Autodesk Inventor part; units mm, degrees
ref_plane "YZ Plane" through (0, 0, 0) normal (1, 0, 0) x (0, 1, 0)
ref_plane "XZ Plane" through (0, 0, 0) normal (0, 1, 0) x (-1, 0, 0)
ref_plane "XY Plane" through (0, 0, 0) normal (0, 0, 1) x (1, 0, 0)
sketch "Sketch1" plane through (0, 0, 0) normal (1, 0, 0) x (0, 1, 0)
  line L0 (0, 0) -> (45.3157, 0)
  line L1 (0, 172.72) -> (163.576, 172.72)
  line L2 (163.576, 172.72) -> (163.576, 198.12)
  line L3 (163.576, 198.12) -> (0, 198.12)
  line L4 (0, 198.12) -> (0, 172.72)
  dimension "d0" = 345.44
  dimension "d1" = 163.576
  dimension "d2" = 25.4
extrude "Extrusion1" add sketch "Sketch1" along normal blind 12.7
sketch "Sketch3" plane through (12.7, 0, 0) normal (1, 0, 0) x (0, 0, -1)
  circle A0 centre (-185.42, 146.05) radius 3.175
  line L0 (-172.72, 0) -> (-172.72, 163.576)
  line L1 (-198.12, 0) -> (-172.72, 0)
  point P0 (0, 0)
  dimension "d10" = 6.35
  dimension "d11" = 12.7
  dimension "d62" = 146.05
extrude "Extrusion3" cut sketch "Sketch3" against normal blind 25.4
chamfer "Chamfer1" distance 9.525 angle 45 1 edges at (6.35, 0, 172.72)
sketch "Sketch4" plane through (12.7, 0, 0) normal (1, 0, 0) x (0, 0, -1)
  circle A0 centre (-185.42, 146.05) radius 3.175
  circle A1 centre (-185.42, 146.05) radius 9.525
  point P0 (0, 0)
  dimension "d18" = 19.05
extrude "Extrusion4" add sketch "Sketch4" along normal blind 19.05
mirror "Mirror2" about plane through (0, 0, 0) normal (0, 0, 1) of "Extrusion1", "Extrusion3", "Chamfer1", "Extrusion4"
sketch "Sketch5" plane through (0, 0, 0) normal (-1, 0, 0) x (0, 0, 1)
  line L0 (172.72, 163.576) -> (198.12, 163.576)
  line L1 (198.12, 163.576) -> (-198.12, 163.576)
  line L2 (-198.12, 163.576) -> (-198.12, 227.076)
  line L3 (-198.12, 227.076) -> (198.12, 227.076)
  line L4 (198.12, 227.076) -> (198.12, 163.576)
  point P0 (0, 0)
  dimension "d21" = 63.5
extrude "Extrusion5" add sketch "Sketch5" against normal up to surface (12.7 mm away)
fillet "Fillet2" radius 25.4 2 edges at (6.35, 227.076, 198.12) (6.35, 227.076, -198.12)
sketch "Sketch6" plane through (12.7, 0, 0) normal (1, 0, 0) x (0, 0, -1)
  line L0 (188.595, 120.65) -> (182.245, 120.65)
  line L1 (179.07, 123.825) -> (179.07, 168.275)
  line L2 (182.245, 171.45) -> (188.595, 171.45)
  line L3 (191.77, 168.275) -> (191.77, 123.825)
  circle A0 centre (185.42, 146.05) radius 3.175
  line L4 (191.77, 120.65) -> (179.07, 171.45) construction
  line L5 (179.07, 120.65) -> (191.77, 171.45) construction
  arc A1 (182.245, 171.45) -> (179.07, 168.275) centre (182.245, 168.275) ccw
  arc A2 (191.77, 168.275) -> (188.595, 171.45) centre (188.595, 168.275) ccw
  arc A3 (188.595, 120.65) -> (191.77, 123.825) centre (188.595, 123.825) ccw
  arc A4 (179.07, 123.825) -> (182.245, 120.65) centre (182.245, 123.825) ccw
  circle A5 centre (185.42, 146.05) radius 9.525
  circle A6 centre (185.42, 165.1) radius 2.6289
  line L6 (185.42, 165.1) -> (185.42, 171.45)
  circle A7 centre (185.42, 127) radius 2.6289
  line L7 (185.42, 127) -> (185.42, 120.65)
  point P0 (0, 0)
  point P1 (191.77, 138.9505)
  point P2 (179.07, 138.9505)
  point P3 (179.07, 153.1495)
  point P4 (191.77, 153.1495)
  dimension "d25" = 12.7
  dimension "d26" = 50.8
  dimension "d27" = 3.175
  dimension "d28" = 5.2578
  dimension "d29" = 6.35
  dimension "d30" = 5.2578
  dimension "d31" = 6.35
extrude "Extrusion6" add sketch "Sketch6" along normal blind 19.05 contours L0 A4 L1 A5 L3 A3 | A5 L1 A1 L2 A2 L3
sketch "Sketch9" plane through (0, 227.076, 172.72) normal (0, 1, 0) x (1, 0, 0)
  line L0 (0, 345.44) -> (0, 0)
  line L1 (0, 228.6) -> (6.35, 228.6)
  line L2 (6.35, 228.6) -> (6.35, 116.84)
  line L3 (6.35, 116.84) -> (12.7, 116.84)
  line L4 (12.7, 345.44) -> (12.7, 0)
  line L5 (0, -25.4) -> (12.7, -25.4)
  point P0 (0, 172.72)
  point P1 (6.35, 172.72)
  point P2 (0, 172.72)
  dimension "d47" = 6.35
  dimension "d48" = 254
sketch "Sketch10" plane through (12.7, 0, 0) normal (1, 0, 0) x (0, 0, -1)
  circle A0 centre (179.07, 17.4625) radius 2.0828
  circle A1 centre (191.77, 48.4187) radius 2.0828
  circle A2 centre (179.07, 79.375) radius 2.0828
  line L0 (185.42, 0) -> (198.12, 0)
  line L1 (198.12, 88.9) -> (198.12, 0)
  line L2 (172.72, 88.9) -> (198.12, 88.9)
  line L3 (172.72, 88.9) -> (172.72, 12.7)
  line L4 (172.72, 12.7) -> (185.42, 0)
  point P0 (0, 0)
  point P1 (-12.7, 88.9)
  dimension "d49" = 6.35
  dimension "d50" = 9.525
  dimension "d51" = 25.4
  dimension "d52" = 76.2
  dimension "d53" = 88.9
  dimension "d54" = 12.7
  dimension "d55" = 4.7625
  dimension "d56" = 6.35
  dimension "d57" = 19.05
  dimension "d58" = 40.4813
  dimension "d59" = 4.1656
extrude "Extrusion8" cut sketch "Sketch10" against normal through all contours A0 | A1 | A2
mirror "Mirror3" about plane through (0, 0, 0) normal (0, 0, 1) of "Extrusion8"
sketch "Sketch11" plane through (31.75, 146.05, 185.42) normal (1, 0, 0) x (0, 0, -1)
  circle A0 centre (0, 0) radius 9.525
  circle A1 centre (0, 0) radius 3.175
  point P0 (185.42, -146.05)
extrude "Extrusion9" cut sketch "Sketch11" against normal up to surface (19.05 mm away)
sketch "Sketch12" plane through (12.7, 0, 0) normal (1, 0, 0) x (0, 0, -1)
  circle A0 centre (-185.42, 146.05) radius 3.175
  line L0 (-185.42, 165.1) -> (-185.42, 127)
  circle A1 centre (-185.42, 165.1) radius 2.6035
  circle A2 centre (-185.42, 127) radius 2.6035
  point P0 (0, 0)
  dimension "d65" = 38.1
  dimension "d66" = 5.207
  dimension "d67" = 5.207
extrude "Extrusion10" cut sketch "Sketch12" against normal blind 25.4 contours A2 | A1
sketch "Sketch13" plane through (0, 0, 0) normal (-1, 0, 0) x (0, 0, 1)
  line L0 (-60.6806, 180.6448) -> (-117.602, 180.6448)
  line L1 (-117.602, 180.6448) -> (-117.602, 215.5698)
  line L2 (-117.602, 215.5698) -> (-60.6806, 215.5698)
  line L3 (-60.6806, 215.5698) -> (-60.6806, 180.6448)
  line L4 (-60.6806, 180.6448) -> (-117.602, 215.5698) construction
  line L5 (-117.602, 180.6448) -> (-60.6806, 215.5698) construction
  line L6 (-198.12, 201.676) -> (-198.12, 0)
  line L7 (-90.0938, 214.5284) -> (-90.0938, 179.6034)
  line L8 (172.72, 227.076) -> (-172.72, 227.076)
  line L9 (-90.0938, 214.5284) -> (-28.448, 214.5284)
  line L10 (-28.448, 214.5284) -> (-28.448, 179.6034)
  line L11 (-28.448, 179.6034) -> (-90.0938, 179.6034)
  line L12 (-90.0938, 179.6034) -> (-90.0938, 214.5284)
  line L13 (-60.6806, 215.5698) -> (4.6736, 215.5698)
  line L14 (4.6736, 215.5698) -> (4.6736, 180.6448)
  line L15 (4.6736, 180.6448) -> (-60.6806, 180.6448)
  line L16 (-60.6806, 180.6448) -> (-60.6806, 215.5698)
  line L17 (-28.448, 214.5284) -> (33.02, 214.5284)
  line L18 (33.02, 214.5284) -> (33.02, 179.6034)
  line L19 (33.02, 179.6034) -> (-28.448, 179.6034)
  line L20 (-28.448, 179.6034) -> (-28.448, 214.5284)
  line L21 (4.6736, 180.6448) -> (62.2808, 180.6448)
  line L22 (62.2808, 180.6448) -> (62.2808, 215.5698)
  line L23 (62.2808, 215.5698) -> (4.6736, 215.5698)
  line L24 (4.6736, 215.5698) -> (4.6736, 180.6448)
  line L25 (33.02, 214.5284) -> (89.535, 214.5284)
  line L26 (89.535, 214.5284) -> (89.535, 179.6034)
  line L27 (89.535, 179.6034) -> (33.02, 179.6034)
  line L28 (33.02, 179.6034) -> (33.02, 214.5284)
  point P0 (0, 0)
  point P1 (-89.1413, 198.1073)
  point P2 (-89.1413, 198.1073)
  dimension "d71" = 80.518
  dimension "d72" = 34.925
  dimension "d74" = 1.0414
  dimension "d75" = 27.5082
  dimension "d76" = 56.9214
  dimension "d77" = 11.5062
  dimension "d78" = 89.154
  dimension "d79" = 65.3542
  dimension "d80" = 61.468
  dimension "d81" = 57.6072
  dimension "d82" = 56.515
hole "Hole1" at (0, 215.5698, -117.602) at (0, 180.6448, -117.602) at (0, 214.5284, -90.0938) at (0, 179.6034, -90.0938) at (0, 180.6448, -60.6806) at (0, 215.5698, -60.6806) at (0, 214.5284, -28.448) at (0, 179.6034, -28.448) at (0, 215.5698, 4.6736) at (0, 180.6448, 4.6736) at (0, 214.5284, 33.02) at (0, 179.6034, 33.02) at (0, 215.5698, 62.2808) at (0, 180.6448, 62.2808) at (0, 179.6034, 89.535) at (0, 214.5284, 89.535) direction (1, 0, 0) diameter 4.445 end through all
sketch "Sketch14" plane through (0, 227.076, 172.72) normal (0, 1, 0) x (1, 0, 0)
  line L0 (0, 345.44) -> (0, 0)
  line L1 (6.35, 245.745) -> (6.35, 99.695)
  line L2 (12.7, 345.44) -> (12.7, 0)
  line L3 (6.35, 99.695) -> (0, 99.695)
  line L4 (0, 0) -> (0, 345.44)
  line L5 (6.35, 245.745) -> (12.7, 245.745)
  point P0 (0, 172.72)
  point P1 (6.35, 172.72)
  point P2 (0, 172.72)
  dimension "d90" = 146.05
equation "\"d30\" = d28"
equation "\"d31\" = d29"
properties part number "Frame"
Verification items for the finished model (mm, model axes). A direction names the side the tool comes from. Coordinates: 2 decimals unless noted, no trailing zeros. Write each loop counter-clockwise with the first axis right and the second up, starting at its lowest first coordinate (ties: lowest second). Pieces come first, ordered by that corner, then holes. Notation, with made-up numbers: (-16.75, 60.5) -> (-1.75, 60.5) arc R22 ccw to (-1.75, 83.5) -> close; hole circle Ø4 at (16, 42). An arc over 180 degrees is marked (long way). One line per item, written item: value. Start each with the question number.
Q1. Cross-section at A-A on y = 64. Enter the section's corners in (x, z).
Q2. Go/stop test with flat-tipped pins: P1, Ø5.5, axis at y = 17.46, z = -179.07, coming from the +X side; P2, Ø2.5, axis at y = 179.6, z = -90.09, coming from the -X side; P3, Ø5, axis at x = 24, z = -186.5, coming from the +Y side; P4, Ø4.5, axis at x = 20.5, y = 158.5, coming from the +Z side. Record where each tip stops, or that it passes through.
Q3. Access from +Z, -Z, +X, -X, +Y, -Y to the whole of each face (thin tool, end or side, straight path). Record for faces 1 (the cylindrical face through (22.092, 145.938, -175.896)), 2 (the cylindrical face through (22.092, 146.162, -194.944)), 3 (the flat face through (6.261, 4.829, -177.416)).
Q4. Cross-section at D-D on x = 4.5. State how many separate pieces and enclosed holes the cut face has, and give its area (3 significant figures).
Q5. Cross-section at C-C on z = 124. Enter the section's corners in (x, y), and give its area (3 significant figures).
Q6. Thickness scan on L1, parallel to Y at x = 7, z = 33; L2, parallel to Y at x = 14, z = -185.42 (3 decimals); L3, parallel to Y at x = 9, z = 185.42 (1 decimal). Record the ranges inside material, lowest first. Write a range as from..to.
Q7. Cross-section at B-B on x = 25. Enter the section's corners in (y, z) (3 decimals), and give its area (3 significant figures).
Checked values:
1. outline: (0, -198.12) -> (12.7, -198.12) -> (12.7, -172.72) -> (0, -172.72) -> close; (0, 172.72) -> (12.7, 172.72) -> (12.7, 198.12) -> (0, 198.12) -> close
2. P1: stops at x = 12.7
2. P2: passes through
2. P3: stops at y = 171.45
2. P4: stops at z = -179.07
3. face 1: +Z, +X
3. face 2: -Z, +X
3. face 3: +X, -X, -Y
4. separate pieces: 1
4. enclosed holes: 26
4. area: 32,700 mm²
5. outline: (0, 163.58) -> (12.7, 163.58) -> (12.7, 227.08) -> (0, 227.08) -> close
5. area: 806 mm²
6. L1: y = 163.58..177.38, 181.83..212.31, 216.75..227.08
6. L2: y = 120.65..124.371, 129.629..142.875, 149.225..162.471, 167.729..171.45
6. L3: y = 0..124.4, 129.6..142.9, 149.2..162.5, 167.7..223.7
7. outline: (120.65, -188.595) arc R3.175 ccw to (123.825, -191.77) -> (138.95, -191.77) arc R9.525 ccw to (153.15, -191.77) -> (168.275, -191.77) arc R3.175 ccw to (171.45, -188.595) -> (171.45, -182.245) arc R3.175 ccw to (168.275, -179.07) -> (153.15, -179.07) arc R9.525 ccw to (138.95, -179.07) -> (123.825, -179.07) arc R3.175 ccw to (120.65, -182.245) -> close; hole circle Ø5.258 at (127, -185.42); hole circle Ø6.35 at (146.05, -185.42); hole circle Ø5.258 at (165.1, -185.42)
7. area: 624 mm²
